```python
from build123d import *

# Parameters (mm, degrees)
SKETCH_1_R      = 1.4
EXTRUDE_1_DEPTH = 1.5
SKETCH_2_W      = 14
SKETCH_2_H      = 13.2
EXTRUDE_2_DEPTH = 6.5
SKETCH_3_W      = 5.6
SKETCH_3_H      = 12.5
EXTRUDE_3_DEPTH = 6
EXTRUDE_3_TAPER = 1
SKETCH_4_W      = 6
SKETCH_4_H      = 8
EXTRUDE_4_DEPTH = 5.7


with BuildPart() as part:
    # 草圖1 → 填料-伸長1 (new body)
    with BuildSketch(Plane.XY):
        with BuildLine():
            Line((25.889258578, 80.943460251), (89.789258578, 80.943460251))
            ThreePointArc((89.789258578, 80.943460251), (91.415604175, 80.269805848), (92.089258578, 78.643460251))
            Line((92.089258578, 78.643460251), (92.089258578, 33.243460251))
            ThreePointArc((92.089258578, 33.243460251), (91.415604175, 31.617114655), (89.789258578, 30.943460251))
            Line((89.789258578, 30.943460251), (25.889258578, 30.943460251))
            ThreePointArc((25.889258578, 30.943460251), (24.262912981, 31.617114655), (23.589258578, 33.243460251))
            Line((23.589258578, 33.243460251), (23.589258578, 78.643460251))
            ThreePointArc((23.589258578, 78.643460251), (24.262912981, 80.269805848), (25.889258578, 80.943460251))
        make_face()
        with Locations((25.939258578, 78.593460251)):
            Circle(SKETCH_1_R, mode=Mode.SUBTRACT)
        with Locations((25.939258578, 33.293460251)):
            Circle(SKETCH_1_R, mode=Mode.SUBTRACT)
        with Locations((89.739258578, 33.293460251)):
            Circle(SKETCH_1_R, mode=Mode.SUBTRACT)
        with Locations((89.739258578, 78.593460251)):
            Circle(SKETCH_1_R, mode=Mode.SUBTRACT)
    extrude(amount=EXTRUDE_1_DEPTH)

    # 草圖2 → 填料-伸長2 (add)
    with BuildSketch(Plane.XY.offset(1.5)):
        with Locations((86.089258578, 45.243460251)):
            Rectangle(SKETCH_2_W, SKETCH_2_H)
    extrude(amount=EXTRUDE_2_DEPTH)

    # 草圖3 → 填料-伸長3 (add)
    with BuildSketch(Plane.XY.offset(1.5)):
        with Locations((73.789258578, 44.693460251)):
            Rectangle(SKETCH_3_W, SKETCH_3_H)
    extrude(amount=EXTRUDE_3_DEPTH, taper=EXTRUDE_3_TAPER)

    # 草圖4 → 填料-伸長4 (add)
    with BuildSketch(Plane.XY.offset(1.5)):
        with Locations((26.589258578, 70.943460251)):
            Rectangle(SKETCH_4_W, SKETCH_4_H)
        with Locations((26.589258578, 40.943460251)):
            Rectangle(SKETCH_4_W, SKETCH_4_H)
    extrude(amount=EXTRUDE_4_DEPTH)


solid = part.part
```
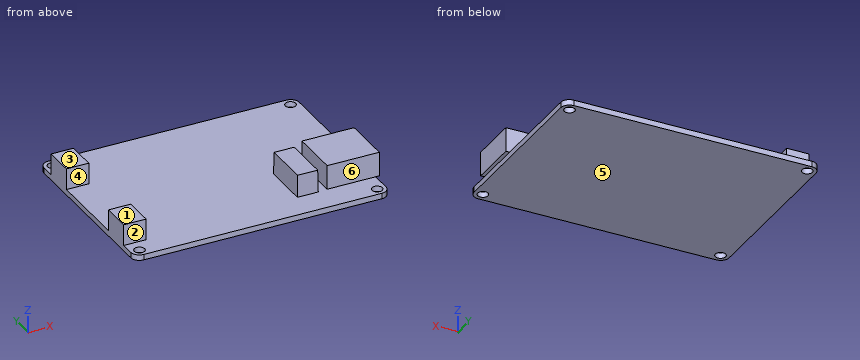
The listing builds one solid part. Answer for the finished solid, in the listing's coordinates (mm). Face numbers are marked on the shaded views. A direction names the side the tool comes from. Round coordinates to 2 decimals unless told otherwise and drop trailing zeros. Loops run counter-clockwise (first coordinate to the right, second up) from the corner with the lowest first, then second, coordinate; pieces in that order, holes last. Notation, with made-up numbers: (44, 28.5) - (91, 28.5) arc R33 ccw to (91, 59.5) - close; hole circle Ø4 at (45, 57.5). An arc over 180 degrees is marked (long way). Return JSON: item names as keys, results as strings. Group by question number.
1. The part is cut by section C-C on y = 49.5. Determine the outline of the cut face in (x, z).
2. The part is cut by section D-D on x = 31. Determine the outline of the cut face in (y, z).
3. Consider probe 1 along X at (y, z) = (50.5, 2); probe 2 along Y at (x, z) = (76, 2.5); probe 3 along Z at (x, y) = (39, 41). Determine where each line is inside the solid, lowest interval first.
4. The part is cut by section A-A on y = 43. Determine the outline of the cut face in (x, z).
5. Each of these flat-tipped pins is pushed along its axis until it touches: P1, Ø5, axis at x = 75.5, y = 36.5, coming from the -Z side; P2, Ø4.5, axis at x = 25, z = 5.5, coming from the -Y side; P3, Ø3, axis at x = 26.5, z = 5, coming from the +Y side; P4, Ø3, axis at y = 48, z = 7, coming from the -X side. Where does it stop, or does it pass through?
6. Which of the six approach directions +Z, -Z, +X, -X, +Y, -Y give full straight-line access (tool end or side, diameter ignored) to the marked faces 1, 2 and 3?
7. The mould has two halves that part along Y. Classify the marked faces 4, 5 and 6: pulls with the +Y half, pulls with the -Y half, needs draft (parallel to the pull), parting line crosses it, or undercut.
8. The part is cut by section B-B on z = 5.75. Determine the outline of the cut face in (x, y).
Resolved:
{
 "1": {"outline": "(23.59, 0) - (92.09, 0) - (92.09, 1.5) - (93.09, 1.5) - (93.09, 8) - (79.09, 8) - (79.09, 1.5) - (76.59, 1.5) - (76.48, 7.5) - (71.09, 7.5) - (70.99, 1.5) - (23.59, 1.5) - close"},
 "2": {"outline": "(30.94, 0) - (80.94, 0) - (80.94, 1.5) - (30.94, 1.5) - close"},
 "3": {"probe 1": "x = 71 to 76.58, 79.09 to 93.09", "probe 2": "y = 38.46 to 50.93", "probe 3": "z = 0 to 1.5"},
 "4": {"outline": "(23.59, 0) - (92.09, 0) - (92.09, 1.5) - (93.09, 1.5) - (93.09, 8) - (79.09, 8) - (79.09, 1.5) - (76.59, 1.5) - (76.48, 7.5) - (71.09, 7.5) - (70.99, 1.5) - (29.59, 1.5) - (29.59, 7.2) - (23.59, 7.2) - close"},
 "5": {"P1": "stops at z = 0", "P2": "stops at y = 36.94", "P3": "stops at y = 74.94", "P4": "stops at x = 71.06"},
 "6": {"face 1": "+Z, -X, +Y, -Y", "face 2": "+Z, +X, -X, -Y", "face 3": "+Z, +X, -X, +Y, -Y"},
 "7": {"face 4": "undercut", "face 5": "needs draft", "face 6": "pulls with the -Y half"},
 "8": {"outline": "(23.59, 36.94) - (29.59, 36.94) - (29.59, 44.94) - (23.59, 44.94) - close; (23.59, 66.94) - (29.59, 66.94) - (29.59, 74.94) - (23.59, 74.94) - close; (71.06, 38.52) - (76.52, 38.52) - (76.52, 50.87) - (71.06, 50.87) - close; (79.09, 38.64) - (93.09, 38.64) - (93.09, 51.84) - (79.09, 51.84) - close"}
}
